Here's how the part is built. I have some questions about the finished solid (model axes, mm). Coordinates: 2 decimals unless noted, no trailing zeros. Write each loop counter-clockwise with the first axis right and the second up, starting at its lowest first coordinate (ties: lowest second). Pieces come first, ordered by that corner, then holes. Notation, with made-up numbers: (-14, -23) - (12, -23) arc R5 cw to (12, -14) - close; hole circle Ø1 at (-23, 69.25). An arc over 180 degrees is marked (long way). Answer in a Markdown table with one row per item. Add a question column.
Item 1: Imagine slicing it at B-B (y = 4.5). Please give me the cut outline in (x, z), plus the area to 3 significant figures.
Item 2: Imagine slicing it at A-A (z = 19). Please give me the cut outline in (x, y), plus the area to 4 significant figures.
Item 3: If I drill on probe 1 along X at (y, z) = (0.8, 5); probe 2 along X at (y, z) = (4.5, 135); probe 3 along Y at (x, z) = (1.5, 257.5), over which ranges is the centre line in solid material (lowest first)? Write a range as from..to.
Item 4: I'm going to push flat-ended pins straight in: pin 1 (6 mm diameter, centred on x = 0.5, z = 105, fed in from +Y); pin 2 (1.9 mm diameter, centred on x = 0, z = 120, fed in from -Y). Where does each tip first touch, or does it pass through?
Item 5: Imagine slicing it at C-C (x = 4.5). Please give me the cut outline in (y, z).
from build123d import *

# Parameters (mm, degrees)
BOSS_EXTRU_1_DEPTH                  = 300
ESQUISSE2_R                         = 1.6
ENL_V_MAT_EXTRU_1_DEPTH             = 301.377366824
F_3_0_3_DURCHMESSER_LANGLOCH1_D     = 3
F_3_0_3_DURCHMESSER_LANGLOCH1_DEPTH = 12.5
F_3_0_3_DURCHMESSER_LANGLOCH1_TIP   = 0.901290929


with BuildPart() as part:
    # Esquisse1 → Boss.-Extru.1 (new body)
    with BuildSketch(Plane.XY):
        Polygon((-11.25, 0), (11.25, 0), (11.25, 10), (9.75, 10), (9.75, 1.5), (-9.75, 1.5), (-9.75, 10), (-11.25, 10), align=None)
    extrude(amount=BOSS_EXTRU_1_DEPTH)

    # Esquisse2 → Enlèv. mat.-Extru.1 (cut, through all)
    with BuildSketch(Plane.XZ):
        with Locations(Location((0, 120, 0), (0, 0, 270))):
            Circle(ESQUISSE2_R)
        with Locations(Location((0, 130, 0), (0, 0, 270))):
            Circle(ESQUISSE2_R)
    extrude(amount=-ENL_V_MAT_EXTRU_1_DEPTH, mode=Mode.SUBTRACT)

    # Ø3.0 (3) Durchmesser Langloch1
    with Locations(Plane(origin=(0, 0, 0), x_dir=(-1, 0, 0), z_dir=(0, -1, 0))):
        with Locations((0, -5)):
            Hole(F_3_0_3_DURCHMESSER_LANGLOCH1_D / 2, depth=F_3_0_3_DURCHMESSER_LANGLOCH1_DEPTH)
            with Locations((0, 0, -(F_3_0_3_DURCHMESSER_LANGLOCH1_DEPTH + F_3_0_3_DURCHMESSER_LANGLOCH1_TIP / 2))):  # 118° drill point
                Cone(0, F_3_0_3_DURCHMESSER_LANGLOCH1_D / 2, F_3_0_3_DURCHMESSER_LANGLOCH1_TIP, mode=Mode.SUBTRACT)


solid = part.part
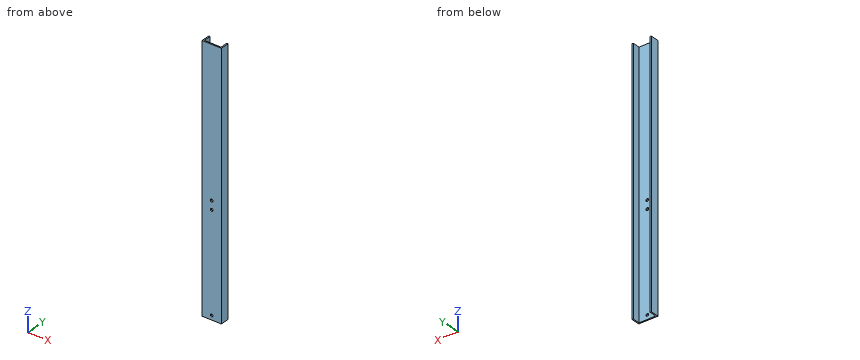
Here are the results:
| question | item | result |
|---|---|---|
| 1 | outline | (-11.25, 0) - (-9.75, 0) - (-9.75, 300) - (-11.25, 300) - close; (9.75, 0) - (11.25, 0) - (11.25, 300) - (9.75, 300) - close |
| 1 | area | 900 mm2 |
| 2 | outline | (-11.25, 0) - (11.25, 0) - (11.25, 10) - (9.75, 10) - (9.75, 1.5) - (-9.75, 1.5) - (-9.75, 10) - (-11.25, 10) - close |
| 2 | area | 59.25 mm2 |
| 3 | probe 1 | x = -11.25..-1.5, 1.5..11.25 |
| 3 | probe 2 | x = -11.25..-9.75, 9.75..11.25 |
| 3 | probe 3 | y = 0..1.5 |
| 4 | pin 1 | stops at y = 1.5 |
| 4 | pin 2 | passes through |
| 5 | outline | (0, 0) - (1.5, 0) - (1.5, 300) - (0, 300) - close |
